Part model, mm, in its own coordinate system. Give positions to 0.01 mm unless a question says otherwise; leave off trailing zeros. Write each loop counter-clockwise with the first axis right and the second up, starting at its lowest first coordinate (ties: lowest second). Pieces come first, ordered by that corner, then holes.
Autodesk Fusion 360 part; units mm, degrees
sketch "Sketch1" plane through (0, 0, 0) normal (0, 0, 1) x (1, 0, 0) in component "Chain Guard"
  line L0 (0, 0) -> (76.2, 0)
  line L1 (76.2, 0) -> (76.2, 25.4)
  line L2 (76.2, 25.4) -> (0, 25.4)
  line L3 (0, 25.4) -> (0, 0)
  line L4 (0, 12.7) -> (76.2, 12.7) construction
  circle A0 centre (19.05, 12.7) radius 3.175
  line L5 (28.575, 9.525) -> (53.975, 9.525)
  arc A1 (53.975, 9.525) -> (53.975, 15.875) centre (53.975, 12.7) ccw
  line L6 (53.975, 15.875) -> (28.575, 15.875)
  arc A2 (28.575, 15.875) -> (28.575, 9.525) centre (28.575, 12.7) ccw
  line L7 (28.575, 12.7) -> (53.975, 12.7) construction
  dimension "d2" = 76.2
  dimension "d3" = 25.4
  dimension "d4" = 6.35
  dimension "d5" = 19.05
  dimension "d6" = 6.35
  dimension "d7" = 28.575
  dimension "d8" = 25.4
extrude "Extrude1" add sketch "Sketch1" along normal blind 2.3114 in component "Chain Guard"
fillet "Fillet1" radius 1.5875 4 edges at (76.2, 0, 1.1557) (76.2, 25.4, 1.1557) (0, 25.4, 1.1557) (0, 0, 1.1557) in component "Chain Guard"
component "Chain Guard" placed x (1, 0, 0) y (0, 1, 0) z (0, 0, 1) at (0, 0, 0)
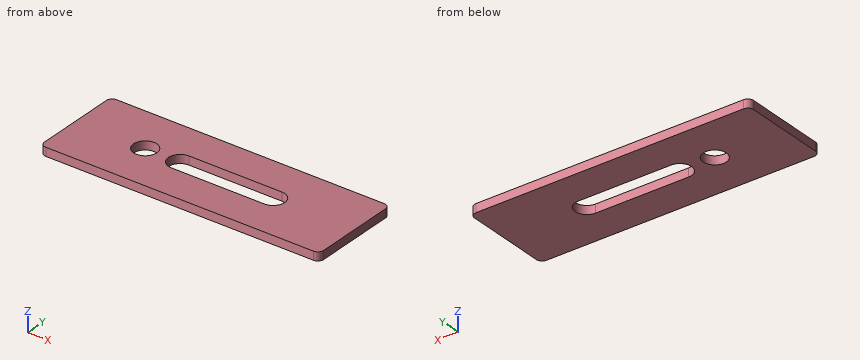
1) Saw through at C-C (x = 19.05). Write the cut outline in (y, z) (3 decimals).
Check result:
outline: (0, 0) - (9.525, 0) - (9.525, 2.311) - (0, 2.311) - close; (15.875, 0) - (25.4, 0) - (25.4, 2.311) - (15.875, 2.311) - close
2) Drill centre lines: L1, parallel to Y at x = 19.05, z = 1.3 (3 decimals); L2, parallel to X at y = 10.75, z = 1.9. Where is each one in solid material? Low to high.
Check result:
L1: y = 0 to 9.525, 15.875 to 25.4
L2: x = 0 to 16.54, 21.56 to 26.07, 56.48 to 76.2
3) Flat gauge pin, fed straight in: P1, Ø1.5, axis at x = 40, y = 15.5, coming from the -Z side. Where does the tip first touch, or does it go through?
Check result:
P1: stops at z = 0
4) Saw through at A-A (y = 12.7). Write the cut outline in (x, z) (3 decimals), and give its area (3 significant figures).
Check result:
outline: (0, 0) - (15.875, 0) - (15.875, 2.311) - (0, 2.311) - close; (22.225, 0) - (25.4, 0) - (25.4, 2.311) - (22.225, 2.311) - close; (57.15, 0) - (76.2, 0) - (76.2, 2.311) - (57.15, 2.311) - close
area: 88.1 mm2
5) Saw through at B-B (z = 0.55). State how many separate pieces and enclosed holes the cut face has, and give its area (3 significant figures).
Check result:
separate pieces: 1
enclosed holes: 2
area: 1,710 mm2
